from build123d import *

# Parameters (mm, degrees)
BOSS_EXTRUDE1_DEPTH      = 10
BOSS_EXTRUDE1_DEPTH_BACK = 10
SKETCH2_R                = 2
CUT_EXTRUDE1_DEPTH       = 10
CUT_EXTRUDE2_DEPTH       = 10


with BuildPart() as part:
    # Sketch1 → Boss-Extrude1 (new, two sides: drawn at the far end of the back side and taken through both)
    with BuildSketch(Plane.XY.offset(-BOSS_EXTRUDE1_DEPTH_BACK)):
        Polygon((0, 0), (0, 16.825), (-3.175, 16.825), (-3.175, -3.175), (16.825, -3.175), (16.825, 0), align=None)
    extrude(amount=BOSS_EXTRUDE1_DEPTH + BOSS_EXTRUDE1_DEPTH_BACK)

    # Sketch2 → Cut-Extrude1 (cut)
    with BuildSketch(Plane(origin=(0, 0, 0), x_dir=(1, 0, 0), z_dir=(0, 1, 0))):
        with Locations(Location((6.825, 0, 0), (0, 0, 270))):
            Circle(SKETCH2_R)
    extrude(amount=-CUT_EXTRUDE1_DEPTH, mode=Mode.SUBTRACT)

    # Sketch3 → Cut-Extrude2 (cut)
    with BuildSketch(Plane(origin=(0, 0, 0), x_dir=(0, 0, -1), z_dir=(1, 0, 0))):
        with BuildLine():
            Line((2, 13.825), (2, 3.825))
            ThreePointArc((2, 3.825), (0, 1.825), (-2, 3.825))
            Line((-2, 3.825), (-2, 13.825))
            ThreePointArc((-2, 13.825), (0, 15.825), (2, 13.825))
        make_face()
    extrude(amount=-CUT_EXTRUDE2_DEPTH, mode=Mode.SUBTRACT)


solid = part.part
Can you work these out from the model? Positions are in its coordinate system, mm. A direction names the side the tool comes from. Give positions to 0.01 mm unless a question says otherwise; leave off trailing zeros. Write each loop counter-clockwise with the first axis right and the second up, starting at its lowest first coordinate (ties: lowest second). Pieces come first, ordered by that corner, then holes. Notation, with made-up numbers: (26, 55) -> (55, 55) arc R18 cw to (55, 88) -> close; hole circle Ø10 at (-39, 15). An arc over 180 degrees is marked (long way). Answer as a JSON object with one key per item and string values. Group by question number.
Item 1: Suppose I cut it at B-B (z = 0). Please give me the cut outline in (x, y) (3 decimals), plus the area to 3 significant figures.
Item 2: Please list where these lines run through material, in increasing order: line 1 (X direction, y = -1.95, z = 0) (3 decimals); line 2 (Z direction, x = -2, y = 5); line 3 (Y direction, x = 14.25, z = 0.5) (3 decimals). Write a range as [from, to].
Item 3: We'd pull the mould along Z, two halves only. Please class faces 1 (the face through (-2, 9, -2)), 2 (the face through (-1, 3, -10)), 3 (the face through (-3.175, 7, -2.4)): +Z half, -Z half, draft (parallel to the pull), parting line (faces both ways), or undercut.
Item 4: Suppose I cut it at D-D (z = -3). Please give me the cut outline in (x, y) (3 decimals).
Item 5: I'm going to push flat-ended pins straight in: P1, Ø4, axis at x = 7, y = 0.5, coming from the -Z side; P2, Ø6, axis at x = 11, y = 3.5, coming from the -Z side; P3, Ø5, axis at x = 9.5, z = 2, coming from the +Y side; P4, Ø3, axis at y = 6.5, z = 1, coming from the +X side. Where does each tip first touch, or does it pass through?
Item 6: For faces 4 (the face through (-1.565, 1.825, -0.044)), 5 (the face through (10, 0, 0)), 6 (the face through (-2, 16.825, 0)), which set-ups out of +Z, -Z, +X, -X, +Y, -Y let a thin tool reach every point of the face, with its end or its side?
Item 7: Suppose I cut it at A-A (x = -1.25). Please give me the cut outline in (y, z) (3 decimals), plus the area to 3 significant figures.
Item 8: Suppose I cut it at C-C (y = 7.25). Please give me the cut outline in (x, z) (3 decimals), plus the area to 3 significant figures.
Findings:
{
 "1": {"outline": "(-3.175, -3.175) -> (4.825, -3.175) -> (4.825, 0) -> (0, 0) -> (0, 1.825) -> (-3.175, 1.825) -> close; (-3.175, 15.825) -> (0, 15.825) -> (0, 16.825) -> (-3.175, 16.825) -> close; (8.825, -3.175) -> (16.825, -3.175) -> (16.825, 0) -> (8.825, 0) -> close", "area": "59.8 mm²"},
 "2": {"line 1": "x = [-3.175, 4.825], [8.825, 16.825]", "line 2": "z = [-10, -2], [2, 10]", "line 3": "y = [-3.175, 0]"},
 "3": {"face 1": "undercut", "face 2": "-Z half", "face 3": "draft"},
 "4": {"outline": "(-3.175, -3.175) -> (16.825, -3.175) -> (16.825, 0) -> (0, 0) -> (0, 16.825) -> (-3.175, 16.825) -> close"},
 "5": {"P1": "stops at z = -10", "P2": "passes through", "P3": "stops at y = 0", "P4": "stops at x = 0"},
 "6": {"face 4": "+X, -X", "face 5": "+Z, -Z, +X, +Y", "face 6": "+Z, -Z, +X, -X, +Y"},
 "7": {"outline": "(-3.175, -10) -> (16.825, -10) -> (16.825, 10) -> (-3.175, 10) -> close; hole (3.825, -2) -> (13.825, -2) arc R2 ccw to (13.825, 2) -> (3.825, 2) arc R2 ccw to start", "area": "347 mm²"},
 "8": {"outline": "(-3.175, -10) -> (0, -10) -> (0, -2) -> (-3.175, -2) -> close; (-3.175, 2) -> (0, 2) -> (0, 10) -> (-3.175, 10) -> close", "area": "50.8 mm²"}
}
